```python
from build123d import *

# Parameters (mm, degrees)
CROQUIS1_R              = 67.5
CROQUIS1_R_2            = 20
SALIENTE_EXTRUIR1_DEPTH = 21
CROQUIS2_R              = 41
CROQUIS2_R_2            = 20
SALIENTE_EXTRUIR2_DEPTH = 4
MATRIZC1_COUNT          = 4


with BuildPart() as part:
    # Croquis1 → Saliente-Extruir1 (new body)
    with BuildSketch(Plane.XY):
        Circle(CROQUIS1_R)
        Circle(CROQUIS1_R_2, mode=Mode.SUBTRACT)
    extrude(amount=SALIENTE_EXTRUIR1_DEPTH)

    # Croquis2 → Saliente-Extruir2 (add)
    with BuildSketch(Plane.XY.offset(21)):
        Circle(CROQUIS2_R)
        Circle(CROQUIS2_R_2, mode=Mode.SUBTRACT)
    extrude(amount=SALIENTE_EXTRUIR2_DEPTH)

    # Croquis7 → Refrentado para perno con cabeza hexagonal de M122 (revolve, cut)
    with BuildSketch(Plane(origin=(0, 34.95, 25), x_dir=(0, -1, 0), z_dir=(1, 0, 0))):
        Polygon((0, 0), (0, 25), (6.5, 25), (6.5, 12.95), (13.89, 12.95), (13.89, 0.025), (13.915, 0), align=None)
    refrentado_para_perno_con_cabeza_hexagon = revolve(axis=Axis((0, 34.95, 31.35), (0, 0, -1)), mode=Mode.SUBTRACT)

    # MatrizC1: Refrentado para perno con cabeza hexagonal de M122 ×4 about axis
    matrizc1_axis = Axis((0, 0, 0), (0, 0, 1))
    for i in range(1, MATRIZC1_COUNT):
        add(refrentado_para_perno_con_cabeza_hexagon.rotate(matrizc1_axis, i * 360 / MATRIZC1_COUNT), mode=Mode.SUBTRACT)


solid = part.part
```
Source: CAD feature listing. Evaluate the final solid. Frame: model axes, mm. A direction names the side the tool comes from. Give positions to 0.01 mm unless a question says otherwise; leave off trailing zeros. Loops run counter-clockwise (first coordinate to the right, second up) from the corner with the lowest first, then second, coordinate; pieces in that order, holes last. Notation, with made-up numbers: (-8.75, 34) - (40.25, 34) arc R12 cw to (40.25, 40) - close; hole circle Ø10 at (31, 1.5). An arc over 180 degrees is marked (long way). Use CSV: the item, a comma, the result in double quotes.
1) Line query: line 1 (Y direction, x = 0, z = 17.75); line 2 (Y direction, x = 1, z = 9.75); line 3 (X direction, y = -4.5, z = 18.75). Output: solid intervals per line, ascending.
Worked out:
line 1,"y = -67.5 to -48.84, -21.06 to -20, 20 to 21.06, 48.84 to 67.5"
line 2,"y = -67.49 to -41.37, -28.53 to -19.97, 19.97 to 28.53, 41.37 to 67.49"
line 3,"x = -67.35 to -48.09, -21.81 to -19.49, 19.49 to 21.81, 48.09 to 67.35"
2) Mould query, pull axis X, two halves, no side actions, for faces 4 (the cylindrical face through (-4.336, -19.524, 12.325)), 5 (the cylindrical face through (-28.81, 29.17, 22.97)), 6 (the cylindrical face through (28.81, -29.17, 22.97)). Classes: +X half, -X half, draft (parallel to the pull), parting line (faces both ways), or undercut.
Worked out:
face 4,"undercut"
face 5,"-X half"
face 6,"+X half"
3) Cut plane C-C (z = 8.25). Output: boundary loops of the cut face in (x, y), and give its area (3 significant figures).
Worked out:
outline,"circle Ø135 at (0, 0); hole circle Ø13 at (-34.95, 0); hole circle Ø40 at (0, 0); hole circle Ø13 at (0, -34.95); hole circle Ø13 at (0, 34.95); hole circle Ø13 at (34.95, 0)"
area,"12,500 mm^2"
4) Pin query (flat end, axial travel): P1, Ø4, axis at x = 12, z = 4.5, coming from the -Y side; P2, Ø4, axis at x = -41.5, y = 32.5, coming from the +Z side; P3, Ø10.5, axis at x = 34.95, y = 0, coming from the -Z side (1 decimal); P4, Ø25, axis at x = -34.95, y = 0, coming from the +Z side. Return the tip coordinate at first contact, or that it passes through.
Worked out:
P1,"stops at y = -66.76"
P2,"stops at z = 21"
P3,"passes through"
P4,"stops at z = 12.05"
5) Cut plane D-D (x = -34.95). Output: boundary loops of the cut face in (y, z) (3 decimals), and give its area (3 significant figures).
Worked out:
outline,"(-57.747, 0) - (-6.5, 0) - (-6.5, 12.05) - (-13.89, 12.05) - (-13.89, 24.975) - (-13.915, 25) - (-21.436, 25) - (-21.436, 21) - (-57.747, 21) - close; (6.5, 0) - (57.747, 0) - (57.747, 21) - (21.436, 21) - (21.436, 25) - (13.915, 25) - (13.89, 24.975) - (13.89, 12.05) - (6.5, 12.05) - close"
area,"2,080 mm^2"
6) Cut plane A-A (y = 0). Output: boundary loops of the cut face in (x, z) (3 decimals).
Worked out:
outline,"(-67.5, 0) - (-41.45, 0) - (-41.45, 12.05) - (-48.84, 12.05) - (-48.84, 21) - (-67.5, 21) - close; (-28.45, 0) - (-20, 0) - (-20, 25) - (-21.035, 25) - (-21.06, 24.975) - (-21.06, 12.05) - (-28.45, 12.05) - close; (20, 0) - (28.45, 0) - (28.45, 12.05) - (21.06, 12.05) - (21.06, 24.975) - (21.035, 25) - (20, 25) - close; (41.45, 0) - (67.5, 0) - (67.5, 21) - (48.84, 21) - (48.84, 12.05) - (41.45, 12.05) - close"
7) Set-up query: faces 1 (the cylindrical face through (-29.17, -28.81, 22.97)), 2 (the flat face through (-3, -41, 12.05)), 3 (the cylindrical face through (28.75, 1.95, 6.11)). Return all of +Z, -Z, +X, -X, +Y, -Y with unobstructed straight access to the full face (end or side cutting, diameter ignored); none if empty.
Worked out:
face 1,"+Z, -X, -Y"
face 2,"+Z"
face 3,"+Z, -Z"
